The model under review builds one solid part; all positions refer to its coordinate system, in mm. A direction names the side the tool comes from. Coordinates: 2 decimals unless noted, no trailing zeros. Order: outer loops, then holes, each group sorted by start corner. A loop starts at its lowest first (then second) coordinate and runs counter-clockwise, first axis right, second up.
```python
from build123d import *

# Parameters (mm, degrees)
SKETCH2_W           = 145
SKETCH2_H           = 90
BOSS_EXTRUDE1_DEPTH = 1.5
SKETCH3_W           = 149
SKETCH3_H           = 94
SKETCH3_W_2         = 145
SKETCH3_H_2         = 90
BOSS_EXTRUDE2_DEPTH = 25
CUT_EXTRUDE1_REACH  = 124.52
SKETCH4_W           = 25
SKETCH4_H           = 15
CUT_EXTRUDE2_REACH  = 160.225
SKETCH5_W           = 18
SKETCH5_H           = 9
SKETCH6_W           = 10
SKETCH6_H           = 5
CUT_EXTRUDE3_DEPTH  = 123.520406464
CUT_EXTRUDE4_REACH  = 160.225
SKETCH7_W           = 15
SKETCH7_H           = 6.5
SKETCH9_W           = 87
SKETCH9_H           = 1
CUT_EXTRUDE5_DEPTH  = 1.5


with BuildPart() as part:
    # Sketch2 → Boss-Extrude1 (new body)
    with BuildSketch(Plane(origin=(0, 0, 0), x_dir=(1, 0, 0), z_dir=(0, 1, 0))):
        Rectangle(SKETCH2_W, SKETCH2_H)
    extrude(amount=BOSS_EXTRUDE1_DEPTH)

    # Sketch3 → Boss-Extrude2 (add)
    with BuildSketch(Plane(origin=(0, 0, 0), x_dir=(1, 0, 0), z_dir=(0, 1, 0))):
        Rectangle(SKETCH3_W, SKETCH3_H)
        Rectangle(SKETCH3_W_2, SKETCH3_H_2, mode=Mode.SUBTRACT)
    extrude(amount=BOSS_EXTRUDE2_DEPTH)

    # Sketch4 → Cut-Extrude1 (cut, up to next)
    with BuildSketch(Plane.XY.offset(47), mode=Mode.PRIVATE) as cut_extrude1_sk1:
        with Locations((-53, 23.5)):
            Rectangle(SKETCH4_W, SKETCH4_H)
    cut_extrude1_tool1 = extrude(cut_extrude1_sk1.sketch, amount=-CUT_EXTRUDE1_REACH, mode=Mode.PRIVATE) & part.part
    add(cut_extrude1_tool1.solids().sort_by_distance((-53, 23.5, 47))[0], mode=Mode.SUBTRACT)

    # Sketch5 → Cut-Extrude2 (cut, up to next)
    with BuildSketch(Plane(origin=(74.5, 0, 0), x_dir=(0, 0, -1), z_dir=(1, 0, 0)), mode=Mode.PRIVATE) as cut_extrude2_sk1:
        with Locations((22, 10.5)):
            Rectangle(SKETCH5_W, SKETCH5_H)
    cut_extrude2_tool1 = extrude(cut_extrude2_sk1.sketch, amount=-CUT_EXTRUDE2_REACH, mode=Mode.PRIVATE) & part.part
    add(cut_extrude2_tool1.solids().sort_by_distance((74.5, 10.5, -22))[0], mode=Mode.SUBTRACT)

    # Sketch6 → Cut-Extrude3 (cut, through all)
    with BuildSketch(Plane.XY.offset(47)):
        with Locations((51.5, 22.5)):
            Rectangle(SKETCH6_W, SKETCH6_H)
    extrude(amount=-CUT_EXTRUDE3_DEPTH, mode=Mode.SUBTRACT)

    # Sketch7 → Cut-Extrude4 (cut, up to next)
    with BuildSketch(Plane.ZY.offset(74.5), mode=Mode.PRIVATE) as cut_extrude4_sk1:
        with Locations((-19.5, 21.75)):
            Rectangle(SKETCH7_W, SKETCH7_H)
    cut_extrude4_tool1 = extrude(cut_extrude4_sk1.sketch, amount=-CUT_EXTRUDE4_REACH, mode=Mode.PRIVATE) & part.part
    add(cut_extrude4_tool1.solids().sort_by_distance((-74.5, 21.75, -19.5))[0], mode=Mode.SUBTRACT)

    # Sketch9 → Cut-Extrude5 (cut)
    with BuildSketch(Plane(origin=(0, 25, 0), x_dir=(1, 0, 0), z_dir=(0, 1, 0))):
        Polygon((-73.5, 12), (-74.5, 12), (-74.5, -47), (-65.5, -47), (-65.5, -46), (-73.5, -46), align=None)
        Polygon((-74.5, 27), (-73.5, 27), (-73.5, 46), (46.5, 46), (46.5, 47), (-74.5, 47), align=None)
        Polygon((56.5, -46), (56.5, -47), (74.5, -47), (74.5, 47), (56.5, 47), (56.5, 46), (73.5, 46), (73.5, -46), align=None)
        with Locations((3, -46.5)):
            Rectangle(SKETCH9_W, SKETCH9_H)
    extrude(amount=-CUT_EXTRUDE5_DEPTH, mode=Mode.SUBTRACT)


solid = part.part
```
(1) We need section D-D, the plane z = 2.5. Write out the cut boundary in (x, y).
A:
outline: (-74.5, 0) - (74.5, 0) - (74.5, 23.5) - (73.5, 23.5) - (73.5, 25) - (72.5, 25) - (72.5, 1.5) - (-72.5, 1.5) - (-72.5, 25) - (-73.5, 25) - (-73.5, 23.5) - (-74.5, 23.5) - close
(2) We need section C-C, the plane y = 8. Write out the cut boundary in (x, z), and give its area (3 significant figures).
A:
outline: (-74.5, -47) - (74.5, -47) - (74.5, -31) - (72.5, -31) - (72.5, -45) - (-72.5, -45) - (-72.5, 45) - (72.5, 45) - (72.5, -13) - (74.5, -13) - (74.5, 47) - (-74.5, 47) - close
area: 920 mm2
(3) Draft analysis for pull direction X (two halves, no side actions). For faces 3 (the face through (-1, 1.5, -1)), 4 (the face through (-72.5, 13, 1)), 5 (the face through (-74.5, 12, 1)), 6 (the face through (-1, 0, -1)), state which applies: released by +X, released by -X, zero draft, split by the parting line, or undercut.
A:
face 3: undercut
face 4: undercut
face 5: released by -X
face 6: zero draft
(4) We need section A-A, the plane z = -22.5. Write out the cut boundary in (x, y), and give its area (3 significant figures).
A:
outline: (-74.5, 0) - (74.5, 0) - (74.5, 6) - (72.5, 6) - (72.5, 1.5) - (-72.5, 1.5) - (-72.5, 18.5) - (-74.5, 18.5) - close; (72.5, 15) - (74.5, 15) - (74.5, 23.5) - (73.5, 23.5) - (73.5, 25) - (72.5, 25) - close
area: 285 mm2
(5) For pin 1 Ø1 at (x, z) = (-53.5, 46) entering from +Y; pin 2 Ø4 at (x, z) = (-52, 20.5) entering from +Y; pin 3 Ø2 at (x, z) = (49.5, -45.5) entering from +Y, all flat-tipped, find the tip position at first contact; note any pin that passes through.
A:
pin 1: stops at y = 16
pin 2: stops at y = 1.5
pin 3: stops at y = 20
(6) Machinability: for faces 1 (the face through (73, 25, 0)), 2 (the face through (-1, 13, 45)), which of the approach directions +Z, -Z, +X, -X, +Y, -Y give a long, thin tool a straight path to every point of the face, cutting with its end or side? Answer none if there is none.
A:
face 1: +Z, -Z, +X, -X, +Y
face 2: +Y
(7) Wall thickness on probe 1 along Z at (x, y) = (-8.5, 9); probe 2 along X at (y, z) = (16, 21); probe 3 along Y at (x, z) = (-54.5, 18): over which ranges is each line inside the solid? List them lowest first.
A:
probe 1: z = -47 to -45, 45 to 47
probe 2: x = -74.5 to -72.5, 72.5 to 74.5
probe 3: y = 0 to 1.5
(8) We need section B-B, the plane x = -55.5. Write out the cut boundary in (y, z), and give its area (4 significant figures).
A:
outline: (0, -47) - (23.5, -47) - (23.5, -46) - (25, -46) - (25, -45) - (1.5, -45) - (1.5, 45) - (16, 45) - (16, 47) - (0, 47) - close
area: 215.5 mm2
